from build123d import *

# Parameters (mm, degrees)
ESQUISSE1_R             = 25
BOSS_EXTRU_1_DEPTH      = 30
COQUE1_T                = -1
ENL_V_START             = -5
ENL_V_MAT_EXTRU_1_DEPTH = 5
ESQUISSE4_W             = 6
ESQUISSE4_H             = 6
ESQUISSE4_R             = 1.5
BOSS_EXTRU_3_DEPTH      = 5


with BuildPart() as part:
    # Esquisse1 → Boss.-Extru.1 (new body)
    with BuildSketch(Plane.XY):
        with BuildLine():
            Line((32.5, 0), (32.5, -45))
            Line((32.5, -45), (17.5, -45))
            Line((17.5, -45), (17.5, -31.622776602))
            ThreePointArc((17.5, -31.622776602), (16.33630621, -29.509890965), (13.928571429, -29.364006844))
            ThreePointArc((13.928571429, -29.364006844), (-27.467513279, 17.371980724), (32.5, 0))
        make_face()
        Circle(ESQUISSE1_R, mode=Mode.SUBTRACT)
    extrude(amount=BOSS_EXTRU_1_DEPTH)

    # Coque1
    coque1_openings = [part.faces().sort_by_distance(p)[0] for p in [
        (25, -45, 15),
        (-25, 0, 15),
    ]]
    offset(amount=COQUE1_T, openings=coque1_openings, kind=Kind.INTERSECTION)

    # Esquisse2 → Enlèv. mat.-Extru.1 (cut)
    with BuildSketch(Plane.XY.offset(30).offset(ENL_V_START)):
        with BuildLine():
            Line((17.5, -31.622776602), (17.5, -45))
            Line((17.5, -45), (32.5, -45))
            Line((32.5, -45), (32.5, 0))
            ThreePointArc((32.5, 0), (-27.467513279, 17.371980724), (13.928571429, -29.364006844))
            ThreePointArc((13.928571429, -29.364006844), (16.33630621, -29.509890965), (17.5, -31.622776602))
        make_face()
    extrude(amount=ENL_V_MAT_EXTRU_1_DEPTH, mode=Mode.SUBTRACT)

    # Esquisse4 → Boss.-Extru.3 (add)
    # profile 1 of 3: a face of its own
    with BuildSketch(Plane(origin=(0, 0, 0), x_dir=(-1, 0, 0), z_dir=(0, 0, -1))):
        with Locations((-35.5, -27)):
            Rectangle(ESQUISSE4_W, ESQUISSE4_H)
        with Locations((-35.5, -27)):
            Circle(ESQUISSE4_R, mode=Mode.SUBTRACT)
    # profile 2 of 3: a face of its own
    with BuildSketch(Plane(origin=(0, 0, 0), x_dir=(-1, 0, 0), z_dir=(0, 0, -1))):
        with BuildLine():
            Line((-24.112106084, 28.692136963), (-20.576572178, 25.156603057))
            ThreePointArc((-20.576572178, 25.156603057), (-18.118767277, 26.980738914), (-15.500260247, 28.5655725))
            Line((-15.500260247, 28.5655725), (-19.869465397, 32.93477765))
            Line((-19.869465397, 32.93477765), (-24.112106084, 28.692136963))
        make_face()
        with Locations((-19.869465397, 28.692136963)):
            Circle(ESQUISSE4_R, mode=Mode.SUBTRACT)
    # profile 3 of 3: a face of its own
    with BuildSketch(Plane(origin=(0, 0, 0), x_dir=(-1, 0, 0), z_dir=(0, 0, -1))):
        with BuildLine():
            Line((19.869465397, 32.93477765), (15.500260247, 28.5655725))
            ThreePointArc((15.500260247, 28.5655725), (18.118767277, 26.980738914), (20.576572178, 25.156603057))
            Line((20.576572178, 25.156603057), (24.112106084, 28.692136963))
            Line((24.112106084, 28.692136963), (19.869465397, 32.93477765))
        make_face()
        with Locations((19.869465397, 28.692136963)):
            Circle(ESQUISSE4_R, mode=Mode.SUBTRACT)
    extrude(amount=-BOSS_EXTRU_3_DEPTH)


solid = part.part
Model file for the job. Use its own axes, mm. A direction names the side the tool comes from. Give positions to 0.01 mm unless a question says otherwise; leave off trailing zeros. Order: outer loops, then holes, each group sorted by start corner. A loop starts at its lowest first (then second) coordinate and runs counter-clockwise, first axis right, second up. Notation, with made-up numbers: (50.5, 48.5) - (60.5, 48.5) arc R13 cw to (60.5, 66.5) - close; hole circle Ø3 at (81, 63). An arc over 180 degrees is marked (long way). Return JSON: item names as keys, results as strings.
1) 3-axis set-ups, long thin cutter, end or side, ignore diameter. For faces 1 (the flat face through (-31.4, -6.1, 25)), 2 (the flat face through (21, 30, 5)), 3 (the flat face through (31.5, -22, 13)), 4 (the flat face through (19, -18, 1)), 5 (the flat face through (-22.02, 30.784, 2.465)): which of +Z, -Z, +X, -X, +Y, -Y reach the whole face in a straight line?
Geometry says:
{"face 1": "+Z, +X, -X, +Y, -Y", "face 2": "+Z, +X, +Y", "face 3": "+Z, -Y", "face 4": "+Z", "face 5": "+Z, -Z, -X, +Y"}
2) Cut at A-A, the plane x = 0. Give the cut face in (y, z).
Geometry says:
{"outline": "(-32.5, 0) - (-25, 0) - (-25, 1) - (-31.5, 1) - (-31.5, 25) - (-32.5, 25) - close; (25, 0) - (32.5, 0) - (32.5, 25) - (31.5, 25) - (31.5, 1) - (25, 1) - close"}
3) Cut at D-D, the plane z = 3. Give the cut face in (x, y).
Geometry says:
{"outline": "(-24.11, 28.69) - (-20.58, 25.16) arc R32.5 ccw to (13.93, -29.36) arc R2.5 cw to (17.5, -31.62) - (17.5, -45) - (18.5, -45) - (18.5, -31.62) arc R3.5 ccw to (13.5, -28.46) arc R31.5 cw (long way) to (31.5, 0) - (31.5, -45) - (32.5, -45) - (32.5, -30) - (38.5, -30) - (38.5, -24) - (32.5, -24) - (32.5, 0) arc R32.5 ccw to (20.58, 25.16) - (24.11, 28.69) - (19.87, 32.93) - (15.5, 28.57) arc R32.5 ccw to (-15.5, 28.57) - (-19.87, 32.93) - close; hole circle Ø3 at (-19.87, 28.69); hole circle Ø3 at (19.87, 28.69); hole circle Ø3 at (35.5, -27)"}
4) Probe line 1 (Y direction, x = 0, z = 0.55); line 2 (Y direction, x = 35.5, z = 1.45); line 3 (X direction, y = 1, z = 19). List the from-to ranges inside material, lowest first. Write a range as from..to.
Geometry says:
{"line 1": "-32.5..-25, 25..32.5", "line 2": "-30..-28.5, -25.5..-24", "line 3": "-32.48..-31.48, 31.48..32.48"}
5) Flat gauge pins, fed straight in: P1, Ø6.5, axis at y = -38.5, z = 14.5, coming from the +X side; P2, Ø6, axis at x = 20, y = 30.5, coming from the +Z side; P3, Ø5, axis at x = 14, z = 18, coming from the +Y side; P4, Ø8, axis at x = -13, y = -11, coming from the +Z side. Where does each tip first touch, or does it go through?
Geometry says:
{"P1": "x = 32.5", "P2": "z = 5", "P3": "y = 30.4", "P4": "through"}
6) Cut at B-B, the plane y = -16. Give the cut face in (x, z).
Geometry says:
{"outline": "(-28.29, 0) - (-19.21, 0) - (-19.21, 1) - (-27.13, 1) - (-27.13, 25) - (-28.29, 25) - close; (19.21, 0) - (32.5, 0) - (32.5, 25) - (31.5, 25) - (31.5, 1) - (19.21, 1) - close"}
7) Pull direction Y, two halves, no side cores. Call faces 6 (the flat face through (32.5, -22, 12)), 7 (the flat face through (22.37, 26.95, 2.46)), 8 (the flat face through (17.654, 30.72, 2.465)): pulls with the +Y half, pulls with the -Y half, needs draft (parallel to the pull), parting line crosses it, or undercut.
Geometry says:
{"face 6": "needs draft", "face 7": "undercut", "face 8": "pulls with the +Y half"}
8) Cut at C-C, the plane x = 35.5. Give the cut face in (y, z), plus the area to 3 significant figures.
Geometry says:
{"outline": "(-30, 0) - (-28.5, 0) - (-28.5, 5) - (-30, 5) - close; (-25.5, 0) - (-24, 0) - (-24, 5) - (-25.5, 5) - close", "area": "15.0 mm²"}
